Part model, mm, in its own coordinate system. A direction names the side the tool comes from. Give positions to 0.01 mm unless a question says otherwise; leave off trailing zeros. Write each loop counter-clockwise with the first axis right and the second up, starting at its lowest first coordinate (ties: lowest second). Pieces come first, ordered by that corner, then holes. Notation, with made-up numbers: M -14,5.5 L 10,5.5 A33 ccw 10,33.5 Z; hole C 34,81.25 d8. An arc over 180 degrees is marked long. Use a Markdown table: item, result.
```python
from build123d import *

# Parameters (mm, degrees)
F1_DEPTH = 12.7
F2_R     = 5.08


# Not quite as in the source:
# - a feature names something its author has since deleted; it is built from what else it names


with BuildPart() as f1:
    # F0 (on Front) → F1 (new body)
    with BuildSketch(Plane.XZ):
        with BuildLine():
            ThreePointArc((-6.6039999947, 74.8653914212), (-31.2484265209, 49.4310412723), (-17.0128613258, 17.0026184017))
            Line((-17.0128613258, 17.0026184017), (17.0128613258, 17.0026184017))
            ThreePointArc((17.0128613258, 17.0026184017), (27.8228399619, 28.5143091682), (31.75, 43.8098011987))
            ThreePointArc((31.75, 43.8098011987), (24.5113290151, 63.9904168958), (6.0960000053, 74.9690900855))
            Line((6.0960000053, 74.9690900855), (6.0960000053, 62.4722737233))
            Line((6.0960000053, 62.4722737233), (6.0960000053, 43.7620282173))
            Line((6.0960000053, 43.7620282173), (-6.6039999947, 43.7620282173))
            Line((-6.6039999947, 43.7620282173), (-6.6039999947, 62.4722737233))
            Line((-6.6039999947, 62.4722737233), (-6.6039999947, 74.8653914212))
        make_face()
        with BuildLine():
            ThreePointArc((17.0128613258, 17.0026184017), (0, 12.0598011987), (-17.0128613258, 17.0026184017))
            Line((-17.0128613258, 17.0026184017), (-17.0128613258, -37.617602489))
            ThreePointArc((-17.0128613258, -37.617602489), (-15.1529893863, -42.1077305495), (-10.6628613258, -43.967602489))
            Line((-10.6628613258, -43.967602489), (10.6628613258, -43.967602489))
            ThreePointArc((10.6628613258, -43.967602489), (15.1529893863, -42.1077305495), (17.0128613258, -37.617602489))
            Line((17.0128613258, -37.617602489), (17.0128613258, 17.0026184017))
        make_face()
        with BuildLine():
            Line((17.0128613258, 17.0026184017), (-17.0128613258, 17.0026184017))
            ThreePointArc((-17.0128613258, 17.0026184017), (0, 12.0598011987), (17.0128613258, 17.0026184017))
        make_face()
    extrude(amount=F1_DEPTH)

    # F2
    f2_edges = [f1.edges().sort_by_distance(p)[0] for p in [
        (6.096, -6.35, 43.762028),
        (-6.604, -6.35, 43.762028),
        (-0.254, 0, 43.762028),
        (-0.254, -12.7, 43.762028),
        (6.096, 0, 59.365559),
        (6.096, -12.7, 59.365559),
        (-6.604, 0, 59.31371),
        (-6.604, -12.7, 59.31371),
    ]]
    fillet(f2_edges, radius=F2_R)


solid = f1.part
```
1. Drill centre lines: L1, parallel to X at y = -3.25, z = -0.5; L2, parallel to Z at x = 0, y = -7; L3, parallel to X at y = -8.5, z = 70. Where is each one in solid material? Low to high.
Findings below:
| item | result |
|---|---|
| L1 | -17.01 to 17.01 |
| L2 | -43.97 to 43.76 |
| L3 | -17.95 to -6.68, 6.17 to 17.95 |
2. Cut at D-D, the plane x = 21.5. Give the cut face in (y, z), then the cut area to 3 significant figures.
Findings below:
| item | result |
|---|---|
| outline | M -12.7,20.45 L 0,20.45 L 0,67.17 L -12.7,67.17 Z |
| area | 593 mm2 |
3. Cut at A-A, the plane z = 55.5. Give the cut face in (x, y).
Findings below:
| item | result |
|---|---|
| outline | M -29.52,-12.7 L -11.68,-12.7 A5.08 ccw -6.6,-7.62 L -6.6,-5.08 A5.08 ccw -11.68,0 L -29.52,0 Z; M 6.1,-7.62 A5.08 ccw 11.18,-12.7 L 29.52,-12.7 L 29.52,0 L 11.18,0 A5.08 ccw 6.1,-5.08 Z |
4. Cut at C-C, the plane z = -9. Give the cut face in (x, y).
Findings below:
| item | result |
|---|---|
| outline | M -17.01,-12.7 L 17.01,-12.7 L 17.01,0 L -17.01,0 Z |
5. Drop flat-ended pins along their axis: P1, Ø2, axis at x = 24.5, y = -10, coming from the +Z side; P2, Ø4, axis at x = -1.5, y = -11, coming from the +Z side; P3, Ø5, axis at y = -10.5, z = -22.5, coming from the +X side. Give the stop position or say it passes through.
Findings below:
| item | result |
|---|---|
| P1 | z = 65.16 |
| P2 | z = 43.58 |
| P3 | x = 17.01 |
6. Two-plate mould, pull along X, no slides. Class faces 5 (the flat face through (0, -12.7, 16)), 6 (the cylindrical face through (-31.15, -6.26, 49.95)), 7 (the cylindrical face through (4.65, -6.37, 45.29)): released by +X, released by -X, zero draft, split by the parting line, or undercut.
Findings below:
| item | result |
|---|---|
| face 5 | zero draft |
| face 6 | released by -X |
| face 7 | undercut |
7. Cut at B-B, the plane y = -3.75. Give the cut face in (x, z), then the cut area to 3 significant figures.
Findings below:
| item | result |
|---|---|
| outline | M -17.01,-37.62 A6.35 ccw -10.66,-43.97 L 10.66,-43.97 A6.35 ccw 17.01,-37.62 L 17.01,17 A31.75 ccw 6.27,74.93 L 6.27,48.84 A5.26 cw 1.02,43.58 L -1.52,43.58 A5.26 cw -6.78,48.84 L -6.78,74.83 A31.75 ccw -17.01,17 Z |
| area | 4,710 mm2 |
8. Tool access for faces 1 (the flat face through (-17.013, -6, -10)), 2 (the cylindrical face through (-0.272, -11.172, 42.313)), 3 (the flat face through (-6.604, -6, 62)), 4 (the flat face through (17.013, -6, -11)): list every direction of +Z, -Z, +X, -X, +Y, -Y with a clear straight run to the whole face (end or side of a thin tool).
Findings below:
| item | result |
|---|---|
| face 1 | -Z, -X, +Y, -Y |
| face 2 | +Z, -Y |
| face 3 | +Z, +Y, -Y |
| face 4 | -Z, +X, +Y, -Y |
